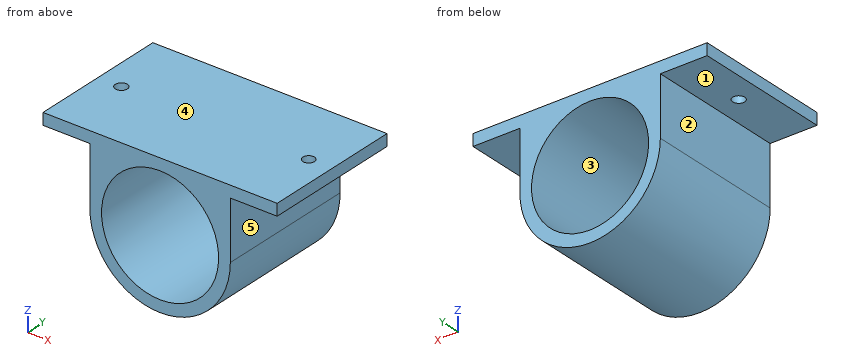
```python
from build123d import *

# Parameters (mm, degrees)
SKETCH1_R           = 31.75
BOSS_EXTRUDE1_DEPTH = 76.2
SKETCH2_R           = 3.2766
SKETCH2_R_2         = 3.175
CUT_EXTRUDE1_DEPTH  = 50.8


with BuildPart() as part:
    # Sketch1 → Boss-Extrude1 (new body)
    with BuildSketch(Plane(origin=(0, 0, 0), x_dir=(1, 0, 0), z_dir=(0, 1, 0))):
        with BuildLine():
            Line((-38.1, -31.75), (-63.5, -31.75))
            Line((-63.5, -31.75), (-63.5, -38.1))
            Line((-63.5, -38.1), (63.5, -38.1))
            Line((63.5, -38.1), (63.5, -31.75))
            Line((63.5, -31.75), (38.1, -31.75))
            Line((38.1, -31.75), (38.1, 0))
            ThreePointArc((38.1, 0), (0, 38.1), (-38.1, 0))
            Line((-38.1, 0), (-38.1, -31.75))
        make_face()
        with Locations(Location((0, 0, 0), (0, 0, 90))):
            Circle(SKETCH1_R, mode=Mode.SUBTRACT)
    extrude(amount=BOSS_EXTRUDE1_DEPTH)

    # Sketch2 → Cut-Extrude1 (cut)
    with BuildSketch(Plane(origin=(0, 0, 31.75), x_dir=(-1, 0, 0), z_dir=(0, 0, -1))):
        with Locations((50.8, 38.1)):
            Circle(SKETCH2_R)
        with Locations((-50.8, 38.1)):
            Circle(SKETCH2_R_2)
    extrude(amount=-CUT_EXTRUDE1_DEPTH, mode=Mode.SUBTRACT)


solid = part.part
```
Here's how the part is built. I have some questions about the finished solid (model axes, mm). Face numbers are marked on the shaded views. A direction names the side the tool comes from. Coordinates: 2 decimals unless noted, no trailing zeros. Order: outer loops, then holes, each group sorted by start corner. A loop starts at its lowest first (then second) coordinate and runs counter-clockwise, first axis right, second up.
1) I need wall thicknesses on line 1 (Y direction, x = 50.8, z = 33.25) (3 decimals); line 2 (X direction, y = 38, z = 34); line 3 (X direction, y = 28, z = -16). Which ranges of each line are inside material? Lowest first, please.
2) Which directions (+Z, -Z, +X, -X, +Y, -Y) give clear straight access to the entire face, cutting with the end or side of a thin tool? Please do the marked faces 4 and 5.
3) Imagine slicing it at C-C on y = 13.5. List the corners of the cut face in (x, z) for me.
4) Imagine slicing it at B-B on x = -50.8. List the corners of the cut face in (y, z) for me, and give its area (3 significant figures).
5) Imagine slicing it at A-A on y = 38.1. List the corners of the cut face in (x, z) for me (3 decimals).
6) We'd pull the mould along Z, two halves only. Please class the marked faces 1, 2 and 3: +Z half, -Z half, draft (parallel to the pull), parting line (faces both ways), or undercut.
7) Imagine slicing it at D-D on z = 25. List the corners of the cut face in (x, y) for me, and give its area (3 significant figures).
8) Will these pins go through, and if not, where does the flat tip stop? pin 1 (12.5 mm diameter, centred on x = -45.5, y = 47.5, fed in from -Z); pin 2 (8.5 mm diameter, centred on x = 50.8, y = 38.1, fed in from +Z); pin 3 (3 mm diameter, centred on y = 34, z = 19, fed in from -X); pin 4 (2 mm diameter, centred on x = 11, y = 63.5, fed in from -Z).
Response values:
1. line 1: y = 0 to 34.925, 41.275 to 76.2
1. line 2: x = -63.5 to -54.08, -47.52 to 47.63, 53.97 to 63.5
1. line 3: x = -34.58 to -27.42, 27.42 to 34.58
2. face 4: +Z, +X, -X, +Y, -Y
2. face 5: -Z, +X, +Y, -Y
3. outline: (-63.5, 31.75) - (-38.1, 31.75) - (-38.1, 0) arc R38.1 ccw to (38.1, 0) - (38.1, 31.75) - (63.5, 31.75) - (63.5, 38.1) - (-63.5, 38.1) - close; hole circle Ø63.5 at (0, 0)
4. outline: (0, 31.75) - (34.82, 31.75) - (34.82, 38.1) - (0, 38.1) - close; (41.38, 31.75) - (76.2, 31.75) - (76.2, 38.1) - (41.38, 38.1) - close
4. area: 442 mm2
5. outline: (-63.5, 31.75) - (-54.077, 31.75) - (-54.077, 38.1) - (-63.5, 38.1) - close; (-47.523, 31.75) - (-38.1, 31.75) - (-38.1, 0) arc R38.1 ccw to (38.1, 0) - (38.1, 31.75) - (47.625, 31.75) - (47.625, 38.1) - (-47.523, 38.1) - close; (53.975, 31.75) - (63.5, 31.75) - (63.5, 38.1) - (53.975, 38.1) - close; hole circle Ø63.5 at (0, 0)
6. face 1: -Z half
6. face 2: draft
6. face 3: undercut
7. outline: (-38.1, 0) - (-19.57, 0) - (-19.57, 76.2) - (-38.1, 76.2) - close; (19.57, 0) - (38.1, 0) - (38.1, 76.2) - (19.57, 76.2) - close
7. area: 2,820 mm2
8. pin 1: stops at z = 31.75
8. pin 2: stops at z = 38.1
8. pin 3: stops at x = -38.1
8. pin 4: stops at z = -36.76
